Read the model definition and answer for the solid it produces. Units are mm, in the model's axes. A direction names the side the tool comes from. Coordinates: 2 decimals unless noted, no trailing zeros. Write each loop counter-clockwise with the first axis right and the second up, starting at its lowest first coordinate (ties: lowest second). Pieces come first, ordered by that corner, then holes.
Item 1: Straight lines are drawn through the part: probe 1 along Y at (x, z) = (-0.3, 0); probe 2 along Z at (x, y) = (-0.25, 37). For each, find the intervals that lie inside material, in ascending order.
Item 2: A tool of negligible diameter and unlimited length cuts with its end or side. For faces 1 (the face through (0, -1, -3)), 2 (the face through (-1, -1, -1)), 3 (the face through (-7.81, 42.04, -1.73)), from which of +Z, -Z, +X, -X, +Y, -Y can it reach the whole face along a straight path? Write none if from no direction.
Item 3: Section B-B (y = 48.5) is taken. Give the vertices of the cut face in (x, z).
Item 4: Determine the mould class of faces 4 (the face through (0.014, -2.14, -1.192)), 5 (the face through (0, -5, 0)), 6 (the face through (-0.01, -4.43, 2.4)) for opening direction Z: released by +Z, released by -Z, zero draft, split by the parting line, or undercut.
Item 5: Section A-A (z = 0) is taken. Give the vertices of the cut face in (x, y), then the cut area to 3 significant figures.
Item 6: Each of these flat-tipped pins is pushed along its axis until it touches: P1, Ø1.6, axis at x = 0, y = -2, coming from the +Z side; P2, Ø5.5, axis at y = -3.5, z = 0.5, coming from the +X side; P3, Ø1.5, axis at x = -1.5, y = 52, coming from the +Z side. Where does it stop, or does it pass through?
from build123d import *

# Parameters (mm, degrees)
SKETCH_1_R          = 9
EXTRUDE_1_DEPTH     = 80
SKETCH_2_R          = 8
CUT_EXTRUDE_1_DEPTH = 77
SKETCH_3_W          = 2
SKETCH_3_H          = 6
EXTRUDE_2_DEPTH     = 5
SKETCH_4_R          = 1.25
CUT_EXTRUDE_2_DEPTH = 5
FILLET_1_R          = 2
FILLET_2_R          = 2
FILLET_3_R          = 2


with BuildPart() as part:
    # 草图1 → 凸台-拉伸1 (new body)
    with BuildSketch(Plane(origin=(0, 0, 0), x_dir=(1, 0, 0), z_dir=(0, 1, 0))):
        with Locations(Location((0, 0, 0), (0, 0, 270))):
            Circle(SKETCH_1_R)
    extrude(amount=EXTRUDE_1_DEPTH)

    # 草图2 → 切除-拉伸1 (cut)
    with BuildSketch(Plane(origin=(0, 80, 0), x_dir=(1, 0, 0), z_dir=(0, 1, 0))):
        with Locations(Location((0, 0, 0), (0, 0, 270))):
            Circle(SKETCH_2_R)
    extrude(amount=-CUT_EXTRUDE_1_DEPTH, mode=Mode.SUBTRACT)

    # 草图3 → 凸台-拉伸2 (add)
    with BuildSketch(Plane(origin=(0, 0, 0), x_dir=(-1, 0, 0), z_dir=(0, -1, 0))):
        Rectangle(SKETCH_3_W, SKETCH_3_H)
    extrude(amount=EXTRUDE_2_DEPTH)

    # 草图4 → 切除-拉伸2 (cut)
    with BuildSketch(Plane(origin=(1, 0, 0), x_dir=(0, 0, -1), z_dir=(1, 0, 0))):
        with Locations((0, -2.515551663)):
            Circle(SKETCH_4_R)
    extrude(amount=-CUT_EXTRUDE_2_DEPTH, mode=Mode.SUBTRACT)

    # 圆角1
    fillet_1_edges = [part.edges().sort_by_distance(p)[0] for p in [
        (0, -5, -3),
    ]]
    fillet(fillet_1_edges, radius=FILLET_1_R)

    # 圆角2
    fillet_2_edges = [part.edges().sort_by_distance(p)[0] for p in [
        (0, -5, 3),
    ]]
    fillet(fillet_2_edges, radius=FILLET_2_R)

    # 圆角3
    fillet_3_edges = [part.edges().sort_by_distance(p)[0] for p in [
        (0, 0, -9),
    ]]
    fillet(fillet_3_edges, radius=FILLET_3_R)


solid = part.part
Established:
1. probe 1: y = -5 to -3.77, -1.27 to 3
1. probe 2: z = -9 to -8, 8 to 9
2. face 1: -Z, +X, -X, -Y
2. face 2: +Z, -Z, -X, -Y
2. face 3: +Y
3. outline: circle Ø18 at (0, 0); hole circle Ø16 at (0, 0)
4. face 4: undercut
4. face 5: zero draft
4. face 6: released by +Z
5. outline: (-9, 2) arc R2 ccw to (-7, 0) - (-1, 0) - (-1, -1.27) - (1, -1.27) - (1, 0) - (7, 0) arc R2 ccw to (9, 2) - (9, 80) - (8, 80) - (8, 3) - (-8, 3) - (-8, 80) - (-9, 80) - close; (-1, -5) - (1, -5) - (1, -3.77) - (-1, -3.77) - close
5. area: 211 mm2
6. P1: stops at z = 3
6. P2: stops at x = 1
6. P3: stops at z = 8.97
